from build123d import *

# Parameters (mm, degrees)
SKETCH1_W           = 40
SKETCH1_H           = 26
BOSS_EXTRUDE1_DEPTH = 15
SKETCH2_R           = 11.5
CUT_EXTRUDE1_DEPTH  = 5
SKETCH3_R           = 5.5
CUT_EXTRUDE2_DEPTH  = 42.243181255
M4_TAPPED_HOLE1_D   = 3.3
M3_TAPPED_HOLE2_D   = 2.5
SKETCH9_W           = 40
SKETCH9_H           = 1
CUT_EXTRUDE4_DEPTH  = 45.452221542


with BuildPart() as part:
    # Sketch1 → Boss-Extrude1 (new, symmetric)
    with BuildSketch(Plane.XY):
        with Locations((0, 13)):
            Rectangle(SKETCH1_W, SKETCH1_H)
    extrude(amount=BOSS_EXTRUDE1_DEPTH, both=True)

    # Sketch2 → Cut-Extrude1 (cut)
    with BuildSketch(Plane.XY.offset(15)):
        with Locations((0, 13)):
            Circle(SKETCH2_R)
    extrude(amount=-CUT_EXTRUDE1_DEPTH, mode=Mode.SUBTRACT)

    # Sketch3 → Cut-Extrude2 (cut, through all)
    with BuildSketch(Plane.XY.offset(10)):
        with Locations((0, 13)):
            Circle(SKETCH3_R)
    extrude(amount=-CUT_EXTRUDE2_DEPTH, mode=Mode.SUBTRACT)

    # M4 Tapped Hole1 (through all)
    with Locations(Plane(origin=(0, 26, 0), x_dir=(1, 0, 0), z_dir=(0, 1, 0))):
        with Locations((-15, 7.5), (15, 7.5), (15, -7.5), (-15, -7.5)):
            Hole(M4_TAPPED_HOLE1_D / 2)

    # M3 Tapped Hole2 (through all)
    with Locations(Plane.XY.offset(10)):
        with Locations((0, 13), (0, 21), (0, 5), (-8, 13), (8, 13)):
            Hole(M3_TAPPED_HOLE2_D / 2)

    # Sketch9 → Cut-Extrude4 (cut, through all)
    with BuildSketch(Plane.XY.offset(15)):
        with Locations((0, 0.5)):
            Rectangle(SKETCH9_W, SKETCH9_H)
    extrude(amount=-CUT_EXTRUDE4_DEPTH, mode=Mode.SUBTRACT)


solid = part.part
Design review of the part built by this model. Coordinates are the model's own, in mm. A direction names the side the tool comes from. Round coordinates to 2 decimals unless told otherwise and drop trailing zeros. Write each loop counter-clockwise with the first axis right and the second up, starting at its lowest first coordinate (ties: lowest second). Pieces come first, ordered by that corner, then holes. Notation, with made-up numbers: (54.5, 57) - (66.5, 57) arc R19 cw to (66.5, 77) - close; hole circle Ø9 at (56.5, 63.5). An arc over 180 degrees is marked (long way). Use a Markdown table: item, result. Add a question column.
1. We need section D-D (x = 0.5). State the section outline as (y, z) points.
2. We need section A-A (z = -7.5). State the section outline as (x, y) points, then the cut area to 3 significant figures.
3. We need section C-C (x = 15). State the section outline as (y, z) points, then the cut area to 3 significant figures.
4. Clearance check with a flat-ended pin moving along its axis: pin 1 (6 mm diameter, centred on x = -6.5, y = 18, fed in from +Z). State where the tip first meets the part, or that it passes through.
5. For faces 5 (the face through (0.27, 19.78, -2.67)), 6 (the face through (-1.5, 24.4, 12.5)), list the 3-axis set-ups (+Z, -Z, +X, -X, +Y, -Y) from which the entire face can be reached by the end or side of a thin tool; tool diameter is ignored.
6. We need section B-B (y = 16). State the section outline as (x, z) points.
7. Mouldability with a two-part tool opening along Z and no side actions: class faces 1 (the face through (8.921, 13.845, -2.675)), 2 (the face through (13.476, 13.325, 8.132)), 3 (the face through (-3, 8, 10)), 4 (the face through (-16.574, 13.325, -7.996)) as +Z half, -Z half, draft (parallel to the pull), parting line (faces both ways), or undercut.
8. Wall thickness on probe 1 along Z at (x, y) = (-15, 12.25); probe 2 along Y at (x, z) = (0, 12.5); probe 3 along Y at (x, z) = (0, 3): over which ranges is each line inside the solid? List them lowest first.
Output:
| question | item | result |
|---|---|---|
| 1 | outline | (1, -15) - (3.85, -15) - (3.85, 10) - (1.51, 10) - (1.51, 15) - (1, 15) - close; (6.15, -15) - (7.52, -15) - (7.52, 10) - (6.15, 10) - close; (18.48, -15) - (19.85, -15) - (19.85, 10) - (18.48, 10) - close; (22.15, -15) - (26, -15) - (26, 15) - (24.49, 15) - (24.49, 10) - (22.15, 10) - close |
| 2 | outline | (-20, 1) - (-16.65, 1) - (-16.65, 26) - (-20, 26) - close; (-13.35, 1) - (13.35, 1) - (13.35, 26) - (-13.35, 26) - close; (16.65, 1) - (20, 1) - (20, 26) - (16.65, 26) - close; hole circle Ø2.5 at (-8, 13); hole circle Ø11 at (0, 13); hole circle Ø2.5 at (0, 5); hole circle Ø2.5 at (0, 21); hole circle Ø2.5 at (8, 13) |
| 2 | area | 720 mm2 |
| 3 | outline | (1, -15) - (26, -15) - (26, -9.15) - (1, -9.15) - close; (1, -5.85) - (26, -5.85) - (26, 5.85) - (1, 5.85) - close; (1, 9.15) - (26, 9.15) - (26, 15) - (1, 15) - close |
| 3 | area | 585 mm2 |
| 4 | pin 1 | stops at z = 10 |
| 5 | face 5 | +Z, -Z |
| 5 | face 6 | +Z |
| 6 | outline | (-20, -15) - (-4.61, -15) - (-4.61, 10) - (-11.1, 10) - (-11.1, 15) - (-20, 15) - close; (4.61, -15) - (20, -15) - (20, 15) - (11.1, 15) - (11.1, 10) - (4.61, 10) - close; hole circle Ø3.3 at (-15, -7.5); hole circle Ø3.3 at (-15, 7.5); hole circle Ø3.3 at (15, -7.5); hole circle Ø3.3 at (15, 7.5) |
| 7 | face 1 | draft |
| 7 | face 2 | undercut |
| 7 | face 3 | +Z half |
| 7 | face 4 | undercut |
| 8 | probe 1 | z = -15 to -9.15, -5.85 to 5.85, 9.15 to 15 |
| 8 | probe 2 | y = 1 to 1.5, 24.5 to 26 |
| 8 | probe 3 | y = 1 to 3.75, 6.25 to 7.5, 18.5 to 19.75, 22.25 to 26 |
